```python
from build123d import *

# Parameters (mm, degrees)
SKETCH2_W          = 2.5
SKETCH2_H          = 3.5
CUT_EXTRUDE1_DEPTH = 3.5
FILLET1_R          = 0.5


with BuildPart() as part:
    # Sketch1 → Revolve1 (revolve)
    with BuildSketch(Plane.XY, mode=Mode.PRIVATE) as revolve1_sk:
        Polygon((0, 7.25), (5, 7.25), (5, 1.25), (8, 1.25), (8, 0), (0, 0), align=None)
    revolve(revolve1_sk.sketch.rotate(Axis((0, 7.25, 0), (0, -1, 0)), 180), axis=Axis((0, 7.25, 0), (0, -1, 0)))

    # Sketch2 → Cut-Extrude1 (cut)
    with BuildSketch(Plane.XZ):
        Rectangle(SKETCH2_W, SKETCH2_H)
    extrude(amount=-CUT_EXTRUDE1_DEPTH, mode=Mode.SUBTRACT)

    # Fillet1
    fillet1_edges = [part.edges().sort_by_distance(p)[0] for p in [
        (5, 7.25, 0),
    ]]
    fillet(fillet1_edges, radius=FILLET1_R)


solid = part.part
```
Check sheet for the modelled part. Datum: model origin and axes. Units: mm. A direction names the side the tool comes from. Round coordinates to 2 decimals unless told otherwise and drop trailing zeros. Order: outer loops, then holes, each group sorted by start corner. A loop starts at its lowest first (then second) coordinate and runs counter-clockwise, first axis right, second up. Notation, with made-up numbers: M -13,47 L 16,47 A20 cw 16,68 Z; hole C 83.5,-33 d5. An arc over 180 degrees is marked long. Answer in a Markdown table with one row per item.
(1) Set-up check for faces 5 (the flat face through (-2, 0, 0)), 6 (the flat face through (1.25, 2, 0)), 7 (the cylindrical face through (5, 4, 0)): record each of +Z, -Z, +X, -X, +Y, -Y from which the full face is reachable in a straight line by a thin tool's end or side.
Findings:
| item | result |
|---|---|
| face 5 | +Z, -Z, +X, -X, -Y |
| face 6 | -Y |
| face 7 | +Y |
(2) Section check B-B on y = 0.5. Record the boundary of the cut face in (x, z).
Findings:
| item | result |
|---|---|
| outline | C 0,0 d16; hole M -1.25,-1.75 L 1.25,-1.75 L 1.25,1.75 L -1.25,1.75 Z |
(3) Gauge pin test, flat ends, axial feed: pin 1 (1.5 mm diameter, centred on y = 4, z = -4.5, fed in from -X); pin 2 (1.5 mm diameter, centred on y = 6.5, z = 0, fed in from +X); pin 3 (1.5 mm diameter, centred on y = 5.5, z = 1.5, fed in from +X). Record the tip position at first contact, or that the pin passes through.
Findings:
| item | result |
|---|---|
| pin 1 | stops at x = -3.31 |
| pin 2 | stops at x = 5 |
| pin 3 | stops at x = 4.94 |
(4) Material ranges on line 1 along Y through (x, z) = (1.75, -7); line 2 along Z through (x, y) = (-0.5, 0.5); line 3 along Z through (x, y) = (-2.25, 6.5), recorded low to high. Write a range as from..to.
Findings:
| item | result |
|---|---|
| line 1 | y = 0..1.25 |
| line 2 | z = -7.98..-1.75, 1.75..7.98 |
| line 3 | z = -4.47..4.47 |
(5) Section check D-D on y = 5.25. Record the boundary of the cut face in (x, z).
Findings:
| item | result |
|---|---|
| outline | C 0,0 d10 |
(6) Section check C-C on x = 0. Record the boundary of the cut face in (y, z).
Findings:
| item | result |
|---|---|
| outline | M 0,-8 L 1.25,-8 L 1.25,-5 L 6.75,-5 A0.5 ccw 7.25,-4.5 L 7.25,4.5 A0.5 ccw 6.75,5 L 1.25,5 L 1.25,8 L 0,8 L 0,1.75 L 3.5,1.75 L 3.5,-1.75 L 0,-1.75 Z |
(7) Draft check along Z on faces 1 (the flat face through (0, 7.25, 0)), 2 (the flat face through (0, 3.5, 0)), 3 (the flat face through (0, 2, 1.75)), 4 (the cylindrical face through (1.73, 0.62, 7.81)). Enter one of: +Z half, -Z half, draft (parallel to the pull), parting line (faces both ways), or undercut.
Findings:
| item | result |
|---|---|
| face 1 | draft |
| face 2 | undercut |
| face 3 | undercut |
| face 4 | parting line |
(8) Section check A-A on z = 0. Record the boundary of the cut face in (x, y).
Findings:
| item | result |
|---|---|
| outline | M -8,0 L -1.25,0 L -1.25,3.5 L 1.25,3.5 L 1.25,0 L 8,0 L 8,1.25 L 5,1.25 L 5,6.75 A0.5 ccw 4.5,7.25 L -4.5,7.25 A0.5 ccw -5,6.75 L -5,1.25 L -8,1.25 Z |
